For this review, use the dimensioned drawing (mm, ordinates from the lowest corner) and the shaded views. Give positions to 0.01 mm unless a question says otherwise; leave off trailing zeros. Order: outer loops, then holes, each group sorted by start corner. A loop starts at its lowest first (then second) coordinate and runs counter-clockwise, first axis right, second up. Notation, with made-up numbers: (43, 5.5) -> (84, 5.5) arc R19 cw to (84, 38.5) -> close; hole circle Ø6 at (50.5, 55). An arc over 180 degrees is marked (long way). One line per item, written item: value. Start each with the question number.
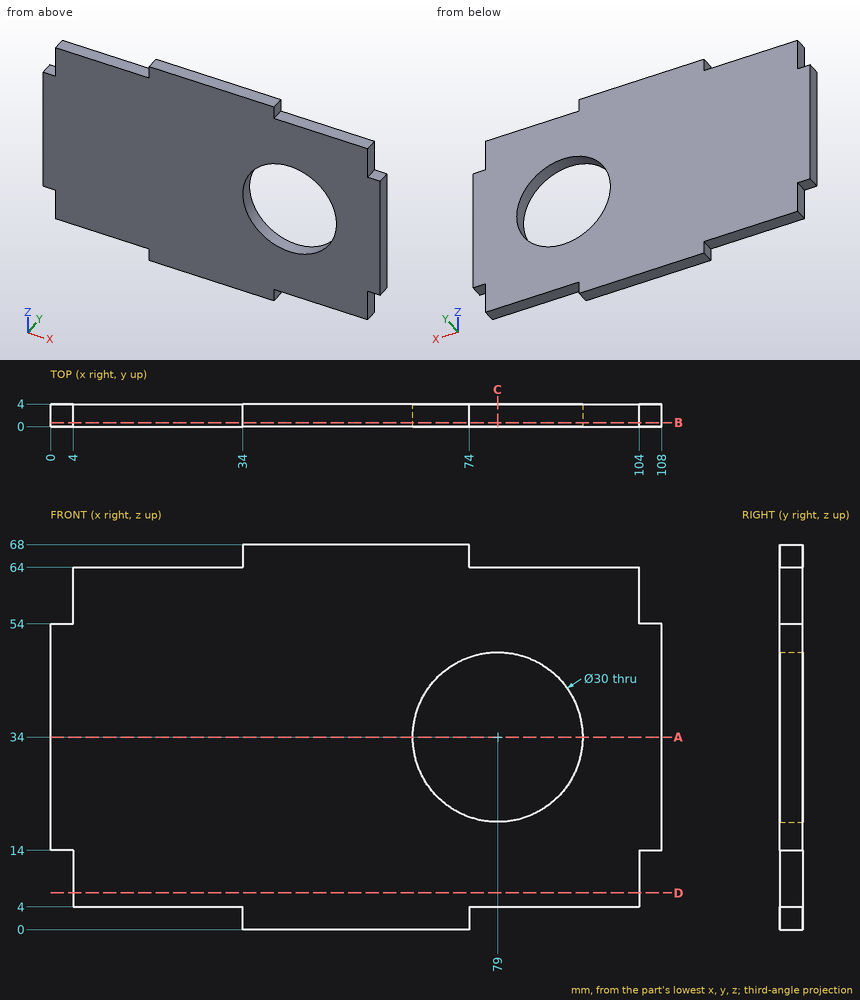
Q1. Take a section at B-B (y = 0.7). State the section outline as (x, z) points, and give its area (3 significant figures).
Q2. For pin 1 Ø1.5 at (x, y) = (19, 3) entering from -Z; pin 2 Ø2 at (x, y) = (1, 3) entering from -Z; pin 3 Ø1.2 at (y, z) = (2.5, 58.5) entering from +X, all flat-tipped, find the tip position at first contact; note any pin that passes through.
Q3. Take a section at C-C (x = 79). State the section outline as (y, z) points.
Q4. Take a section at A-A (z = 34). State the section outline as (x, y) points.
Q5. For line 1 along X through (y, z) = (1.1, 34); line 2 along Z through (x, y) = (79, 1.8); line 3 along X through (y, z) = (1.9, 6.5), list the stretches that pass through material, from the lowest coordinate up.
Q6. Take a section at D-D (z = 6.5). State the section outline as (x, y) points, and give its area (3 significant figures).
Answers below:
1. outline: (0, 14) -> (4, 14) -> (4, 4) -> (34, 4) -> (34, 0) -> (74, 0) -> (74, 4) -> (104, 4) -> (104, 14) -> (108, 14) -> (108, 54) -> (104, 54) -> (104, 64) -> (74, 64) -> (74, 68) -> (34, 68) -> (34, 64) -> (4, 64) -> (4, 54) -> (0, 54) -> close; hole circle Ø30 at (79, 34)
1. area: 5,930 mm²
2. pin 1: stops at z = 4
2. pin 2: stops at z = 14
2. pin 3: stops at x = 104
3. outline: (0, 4) -> (4, 4) -> (4, 19) -> (0, 19) -> close; (0, 49) -> (4, 49) -> (4, 64) -> (0, 64) -> close
4. outline: (0, 0) -> (64, 0) -> (64, 4) -> (0, 4) -> close; (94, 0) -> (108, 0) -> (108, 4) -> (94, 4) -> close
5. line 1: x = 0 to 64, 94 to 108
5. line 2: z = 4 to 19, 49 to 64
5. line 3: x = 4 to 104
6. outline: (4, 0) -> (104, 0) -> (104, 4) -> (4, 4) -> close
6. area: 400 mm²
